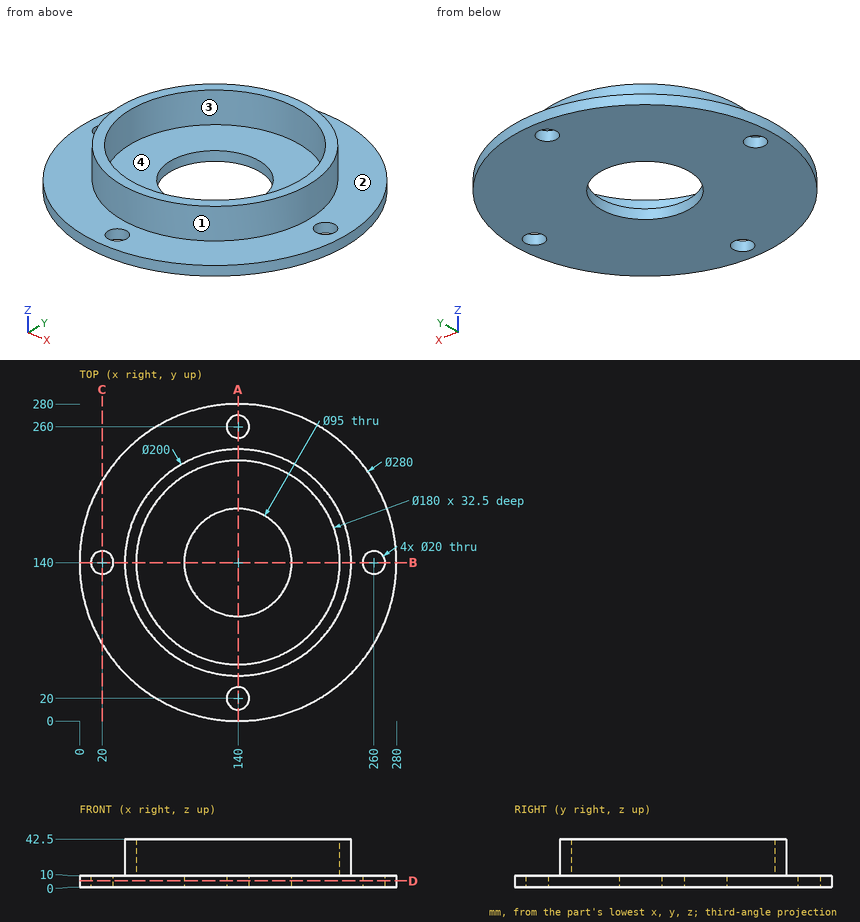
Check sheet for the drawn part. Datum: minimum x, y, z corner. Units: mm. Give positions to 0.01 mm unless a question says otherwise; leave off trailing zeros. Order: outer loops, then holes, each group sorted by start corner. A loop starts at its lowest first (then second) coordinate and runs counter-clockwise, first axis right, second up. Notation, with made-up numbers: (83.25, 38) -> (136.25, 38) arc R13 ccw to (136.25, 43) -> close; hole circle Ø1 at (-9, 16.5). An arc over 180 degrees is marked (long way). Answer as CSV lines item,"result".
Q1. Sectioned sample at C-C on x = 20. Record the cut outline in (y, z).
Solutions:
outline,"(67.89, 0) -> (130, 0) -> (130, 10) -> (67.89, 10) -> close; (150, 0) -> (212.11, 0) -> (212.11, 10) -> (150, 10) -> close"
Q2. Scan lines: probe 1 along Y at (x, z) = (140, 2); probe 2 along Z at (x, y) = (251, 149); probe 3 along X at (y, z) = (141, 13.5) (3 decimals). Record each from-to range of solid material in increasing order.
Solutions:
probe 1,"y = 0 to 10, 30 to 92.5, 187.5 to 250, 270 to 280"
probe 2,"z = 0 to 10"
probe 3,"x = 40.005 to 50.006, 229.994 to 239.995"
Q3. Depth check by flat-ended pin: pin 1 (5 mm diameter, centred on y = 69, z = 35.5, fed in from +X); pin 2 (2 mm diameter, centred on y = 171, z = 18.5, fed in from -X); pin 3 (12 mm diameter, centred on x = 185.5, z = 24.5, fed in from +Y); pin 4 (16 mm diameter, centred on x = 140, y = 20, fed in from +Z). Enter the tip coordinate at first touch or a pass-through.
Solutions:
pin 1,"stops at x = 212.85"
pin 2,"stops at x = 44.61"
pin 3,"stops at y = 231.87"
pin 4,"passes through"
Q4. Sectioned sample at A-A on x = 140. Record the cut outline in (y, z), plus the area to 3 significant figures.
Solutions:
outline,"(0, 0) -> (10, 0) -> (10, 10) -> (0, 10) -> close; (30, 0) -> (92.5, 0) -> (92.5, 10) -> (50, 10) -> (50, 42.5) -> (40, 42.5) -> (40, 10) -> (30, 10) -> close; (187.5, 0) -> (250, 0) -> (250, 10) -> (240, 10) -> (240, 42.5) -> (230, 42.5) -> (230, 10) -> (187.5, 10) -> close; (270, 0) -> (280, 0) -> (280, 10) -> (270, 10) -> close"
area,"2,100 mm²"
Q5. Sectioned sample at D-D on z = 5.5. Record the cut outline in (x, y), plus the area to 3 significant figures.
Solutions:
outline,"circle Ø280 at (140, 140); hole circle Ø20 at (20, 140); hole circle Ø95 at (140, 140); hole circle Ø20 at (140, 20); hole circle Ø20 at (140, 260); hole circle Ø20 at (260, 140)"
area,"53,200 mm²"
Q6. Release check for a two-part mould opening along X. For the marked faces 1, 2, 3 and 4 record: +X half, -X half, draft (parallel to the pull), parting line (faces both ways), or undercut.
Solutions:
face 1,"parting line"
face 2,"draft"
face 3,"undercut"
face 4,"undercut"
